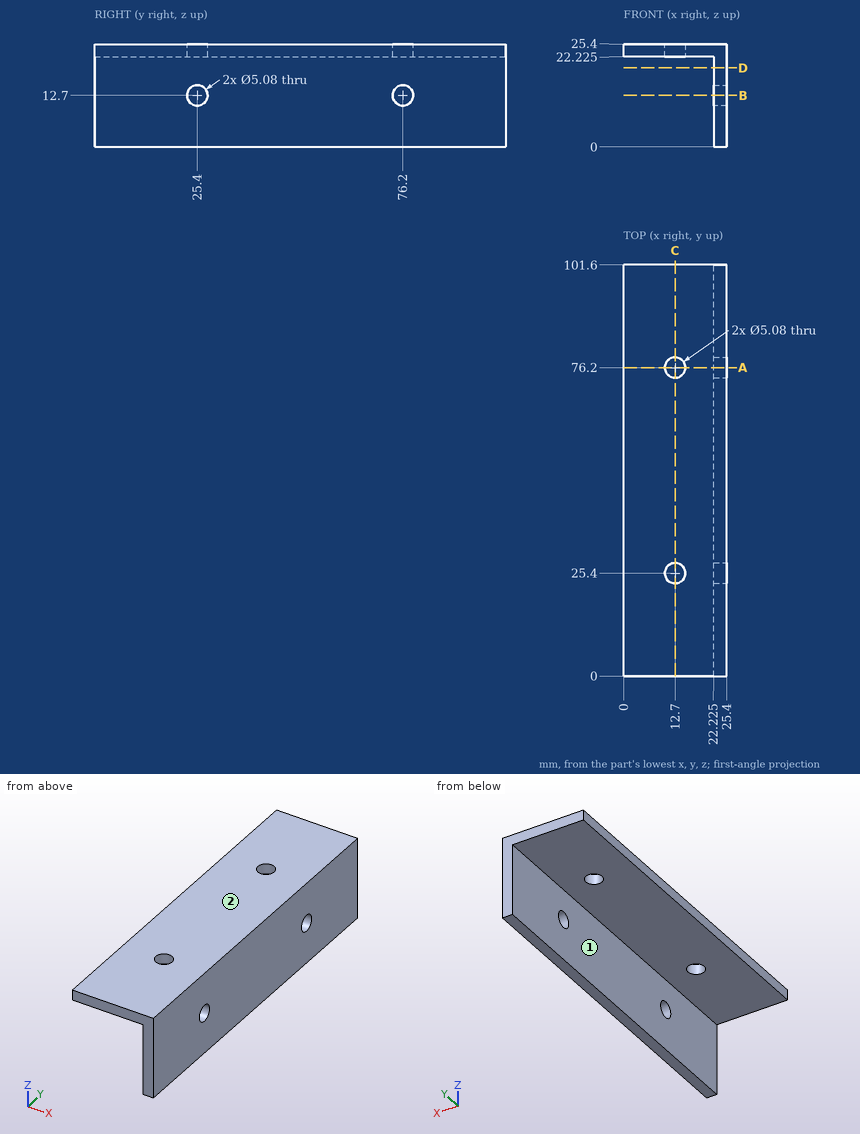
Study the drawing (mm; zero at the part's minimum x, y, z) and answer. A direction names the side the tool comes from. Give positions to 0.01 mm unless a question says otherwise; leave off trailing zeros. Write each loop counter-clockwise with the first axis right and the second up, starting at its lowest first coordinate (ties: lowest second). Pieces come first, ordered by that corner, then holes. Notation, with made-up numbers: M 24.25,-16.75 L 51.25,-16.75 A10 cw 51.25,-0.75 Z; hole C 63,60 d5. An arc over 180 degrees is marked long. Put each result on its own line as item: value. Start each with the question number.
1. Which of the six approach directions +Z, -Z, +X, -X, +Y, -Y give full straight-line access (tool end or side, diameter ignored) to the marked faces 1 and 2?
2. The part is cut by section C-C, the plane x = 12.7. Give the vertices of the cut face in (y, z) (3 decimals).
3. The part is cut by section B-B, the plane z = 12.7. Give the vertices of the cut face in (x, y) (3 decimals).
4. Consider line 1 along Y through (x, z) = (12.7, 23.35); line 2 along X through (y, z) = (25.4, 24.65). Determine where each line is inside the solid, lowest interval first.
5. The part is cut by section D-D, the plane z = 19.5. Give the vertices of the cut face in (x, y) (3 decimals).
6. Each of these flat-tipped pins is pushed along its axis until it touches: pin 1 Ø4 at (x, z) = (15.5, 20.5) entering from +Y; pin 2 Ø6 at (y, z) = (76.2, 12.7) entering from -X (3 decimals); pin 3 Ø3 at (y, z) = (25.4, 12.7) entering from -X; pin 4 Ø10 at (x, y) = (15.5, 57) entering from -Z (3 decimals). Where does it stop, or does it pass through?
7. The part is cut by section A-A, the plane y = 76.2. Give the vertices of the cut face in (x, z) (3 decimals).
Final values:
1. face 1: -Z, -X, +Y, -Y
1. face 2: +Z, +X, -X, +Y, -Y
2. outline: M 0,22.225 L 22.86,22.225 L 22.86,25.4 L 0,25.4 Z; M 27.94,22.225 L 73.66,22.225 L 73.66,25.4 L 27.94,25.4 Z; M 78.74,22.225 L 101.6,22.225 L 101.6,25.4 L 78.74,25.4 Z
3. outline: M 22.225,0 L 25.4,0 L 25.4,22.86 L 22.225,22.86 Z; M 22.225,27.94 L 25.4,27.94 L 25.4,73.66 L 22.225,73.66 Z; M 22.225,78.74 L 25.4,78.74 L 25.4,101.6 L 22.225,101.6 Z
4. line 1: y = 0 to 22.86, 27.94 to 73.66, 78.74 to 101.6
4. line 2: x = 0 to 10.16, 15.24 to 25.4
5. outline: M 22.225,0 L 25.4,0 L 25.4,101.6 L 22.225,101.6 Z
6. pin 1: stops at y = 101.6
6. pin 2: stops at x = 22.225
6. pin 3: passes through
6. pin 4: stops at z = 22.225
7. outline: M 0,22.225 L 10.16,22.225 L 10.16,25.4 L 0,25.4 Z; M 15.24,22.225 L 22.225,22.225 L 22.225,15.24 L 25.4,15.24 L 25.4,25.4 L 15.24,25.4 Z; M 22.225,0 L 25.4,0 L 25.4,10.16 L 22.225,10.16 Z
